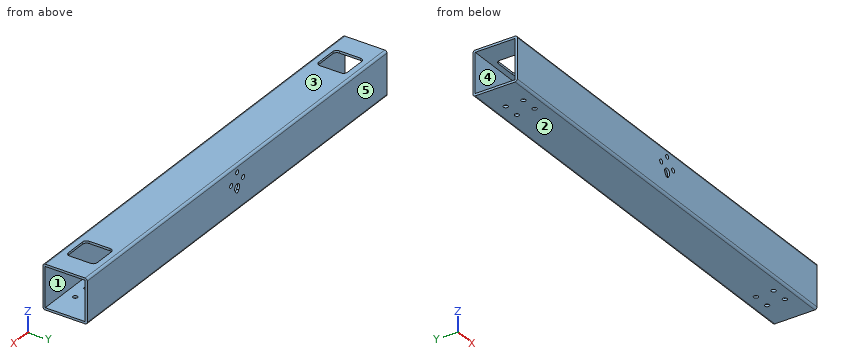
from build123d import *

# Parameters (mm, degrees)
SKETCH022_W             = 36
SKETCH022_H             = 36
PAD020_DEPTH            = 400
SKETCH023_R             = 3.395011
POCKET002_DEPTH         = 40
SKETCH024_R             = 2
POCKET003_DEPTH         = 25
POCKET004_DEPTH         = 5
SKETCH026_R             = 2
POCKET005_DEPTH         = 40
POCKET006_DEPTH         = 50
BODY018_PLACEMENT_ANGLE = 270


with BuildPart() as part:
    # Sketch022 → Pad020 (new body)
    with BuildSketch(Plane.XZ):
        with BuildLine():
            Line((0, -2), (0, -38))
            ThreePointArc((0, -38), (0.585786, -39.414214), (2, -40))
            Line((2, -40), (38, -40))
            ThreePointArc((38, -40), (39.414214, -39.414214), (40, -38))
            Line((40, -38), (40, -2))
            ThreePointArc((40, -2), (39.414214, -0.585786), (38, 0))
            Line((38, 0), (2, 0))
            ThreePointArc((2, 0), (0.585786, -0.585786), (0, -2))
        make_face()
        with Locations((20, -20)):
            Rectangle(SKETCH022_W, SKETCH022_H, mode=Mode.SUBTRACT)
    extrude(amount=PAD020_DEPTH)

    # Sketch023 (on Face1 of Pad020) → Pocket002 (cut)
    with BuildSketch(Plane(origin=(0, 0, 0), x_dir=(0, 0, -1), z_dir=(-1, 0, 0))):
        with Locations((20, 200)):
            Circle(SKETCH023_R)
    extrude(amount=-POCKET002_DEPTH, mode=Mode.SUBTRACT)

    # Sketch024 (on Face13 of Pocket002) → Pocket003 (cut, symmetric)
    with BuildSketch(Plane(origin=(0, 0, -38), x_dir=(-1, 0, 0), z_dir=(0, 0, 1))):
        with Locations((-28.25, 359.5)):
            Circle(SKETCH024_R)
        with Locations((-12.217429, 359.5)):
            Circle(SKETCH024_R)
        with Locations((-12.217429, 374.5)):
            Circle(SKETCH024_R)
        with Locations((-28.20008, 374.5)):
            Circle(SKETCH024_R)
        with Locations((-28.25, 40.5)):
            Circle(SKETCH024_R)
        with Locations((-12.217429, 40.5)):
            Circle(SKETCH024_R)
        with Locations((-12.217429, 25.5)):
            Circle(SKETCH024_R)
        with Locations((-28.20008, 25.5)):
            Circle(SKETCH024_R)
    extrude(amount=POCKET003_DEPTH, both=True, mode=Mode.SUBTRACT)

    # Sketch025 (on Face7 of Pocket003) → Pocket004 (cut)
    with BuildSketch(Plane(origin=(0, 0, 0), x_dir=(-1, 0, 0), z_dir=(0, 0, 1))):
        with BuildLine():
            Line((-33, 376.5), (-33, 357.5))
            ThreePointArc((-33, 357.5), (-31.974874, 355.025126), (-29.5, 354))
            Line((-29.5, 354), (-10.5, 354))
            ThreePointArc((-10.5, 354), (-8.025126, 355.025126), (-7, 357.5))
            Line((-7, 357.5), (-7, 376.5))
            ThreePointArc((-7, 376.5), (-8.025126, 378.974874), (-10.5, 380))
            Line((-10.5, 380), (-29.5, 380))
            ThreePointArc((-29.5, 380), (-31.974874, 378.974874), (-33, 376.5))
        make_face()
        with BuildLine():
            Line((-33, 23.5), (-33, 42.5))
            ThreePointArc((-29.5, 46), (-31.974874, 44.974874), (-33, 42.5))
            Line((-29.5, 46), (-10.5, 46))
            ThreePointArc((-7, 42.5), (-8.025126, 44.974874), (-10.5, 46))
            Line((-7, 42.5), (-7, 23.5))
            ThreePointArc((-10.5, 20), (-8.025126, 21.025126), (-7, 23.5))
            Line((-10.5, 20), (-29.5, 20))
            ThreePointArc((-33, 23.5), (-31.974874, 21.025126), (-29.5, 20))
        make_face()
    extrude(amount=-POCKET004_DEPTH, mode=Mode.SUBTRACT)

    # Sketch026 (on Face10 of Pocket004) → Pocket005 (cut)
    with BuildSketch(Plane(origin=(40, 0, 0), x_dir=(0, 0, 1), z_dir=(1, 0, 0))):
        with Locations((-14.500015, 192)):
            Circle(SKETCH026_R)
        with Locations((-14.499969, 208)):
            Circle(SKETCH026_R)
        with Locations((-6.5, 200)):
            Circle(SKETCH026_R)
        with Locations((-22.5, 200)):
            Circle(SKETCH026_R)
    extrude(amount=-POCKET005_DEPTH, mode=Mode.SUBTRACT)

    # Sketch026 (on Face10 of Pocket004) → Pocket006 (cut)
    with BuildSketch(Plane(origin=(40, 0, 0), x_dir=(0, 0, 1), z_dir=(1, 0, 0))):
        with Locations((-14.500015, 192)):
            Circle(SKETCH026_R)
        with Locations((-14.499969, 208)):
            Circle(SKETCH026_R)
        with Locations((-6.5, 200)):
            Circle(SKETCH026_R)
        with Locations((-22.5, 200)):
            Circle(SKETCH026_R)
    extrude(amount=-POCKET006_DEPTH, mode=Mode.SUBTRACT)


with BuildPart() as part_1:
    # Body018 placement: moved
    add(part.part.moved(Location((386, -140.983559, 55))).rotate(Axis((386, -140.983559, 55), (0, 0, 1)), BODY018_PLACEMENT_ANGLE))


solid = part_1.part
Verification items for the finished model (mm, model axes). Face numbers are marked on the shaded views. A direction names the side the tool comes from. Give positions to 0.01 mm unless a question says otherwise; leave off trailing zeros. Write each loop counter-clockwise with the first axis right and the second up, starting at its lowest first coordinate (ties: lowest second). Pieces come first, ordered by that corner, then holes. Notation, with made-up numbers: M -27.5,-23.5 L 15.5,-23.5 A29 ccw 15.5,13.5 Z; hole C 85,76.5 d7. An arc over 180 degrees is marked long. Put each result on its own line as item: value. Start each with the question number.
1. Set-up check for the marked faces 4 and 5: record each of +Z, -Z, +X, -X, +Y, -Y from which the full face is reachable in a straight line by a thin tool's end or side.
2. Draft check along Z on the marked faces 1, 2 and 3. Enter one of: +Z half, -Z half, draft (parallel to the pull), parting line (faces both ways), or undercut.
3. Section check A-A (y = -159.5). Record the cut outline in (x, z), and give its area (3 significant figures).
4. Scan lines: line 1 along Z through (x, y) = (365, -143.5); line 2 along Y through (x, z) = (228, 19); line 3 along Z through (x, y) = (186, -179.95). Record each from-to range of solid material in increasing order. Write a range as [from, to].
5. Go/stop test with flat-tipped pins: pin 1 Ø0.6 at (x, z) = (355.5, 53.5) entering from +Y; pin 2 Ø5 at (x, y) = (11.5, -169.18) entering from +Z; pin 3 Ø0.6 at (x, z) = (14.5, 54) entering from +Y; pin 4 Ø3 at (x, y) = (11.5, -153.2) entering from -Z. Record where each tip stops, or that it passes through.
6. Section check C-C (x = 121). Record the cut outline in (y, z).
7. Section check B-B (z = 21.5). Record the cut outline in (x, y).
Answer list:
1. face 4: +X, -X
1. face 5: +Z, -Z, +X, -X, +Y
2. face 1: undercut
2. face 2: -Z half
2. face 3: +Z half
3. outline: M -14,15 L 386,15 L 386,17 L -14,17 Z; M -14,53 L 6,53 L 6,55 L -14,55 Z; M 32,53 L 340,53 L 340,55 L 32,55 Z; M 366,53 L 386,53 L 386,55 L 366,55 Z
3. area: 1,500 mm2
4. line 1: [15, 17], [53, 55]
4. line 2: [-180.98, -178.98], [-142.98, -140.98]
4. line 3: [15.25, 30.5], [38.4, 46.5], [50.5, 54.75]
5. pin 1: y = -140.99
5. pin 2: z = 17
5. pin 3: y = -141.11
5. pin 4: through
6. outline: M -180.98,17 A2 ccw -178.98,15 L -142.98,15 A2 ccw -140.98,17 L -140.98,53 A2 ccw -142.98,55 L -178.98,55 A2 ccw -180.98,53 Z; hole M -178.98,17 L -142.98,17 L -142.98,53 L -178.98,53 Z
7. outline: M -14,-180.98 L 386,-180.98 L 386,-178.98 L -14,-178.98 Z; M -14,-142.98 L 386,-142.98 L 386,-140.98 L -14,-140.98 Z
